The model under review builds one solid part; all positions refer to its coordinate system, in mm. Give positions to 0.01 mm unless a question says otherwise; leave off trailing zeros. Write each loop counter-clockwise with the first axis right and the second up, starting at its lowest first coordinate (ties: lowest second). Pieces come first, ordered by that corner, then holes. Notation, with made-up numbers: M 75,62 L 128,62 A14 cw 128,82 Z; hole C 83.25,72 d10. An arc over 180 degrees is marked long. Write item = value, one per line. Start each with the question number.
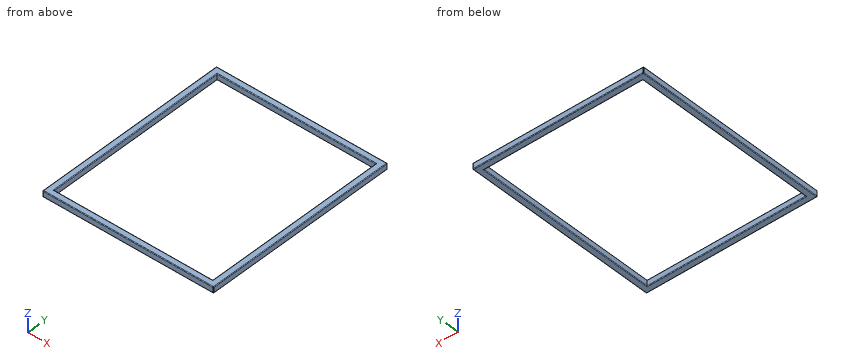
```python
from build123d import *

# Parameters (mm, degrees)
SKETCH1_W           = 711.2
SKETCH1_H           = 812.8
SKETCH1_W_2         = 660.4
SKETCH1_H_2         = 762
BOSS_EXTRUDE1_DEPTH = 25.4
FILLET1_R           = 2.54


with BuildPart() as part:
    # Sketch1 → Boss-Extrude1 (new body)
    with BuildSketch(Plane.XY):
        with Locations((-355.6, 406.4)):
            Rectangle(SKETCH1_W, SKETCH1_H)
        with Locations((-355.6, 406.4)):
            Rectangle(SKETCH1_W_2, SKETCH1_H_2, mode=Mode.SUBTRACT)
    extrude(amount=BOSS_EXTRUDE1_DEPTH)

    # Fillet1
    fillet1_edges = [part.edges().sort_by_distance(p)[0] for p in [
        (-711.2, 406.4, 25.4),
        (-25.4, 406.4, 0),
        (-355.6, 787.4, 0),
        (-685.8, 406.4, 0),
        (-355.6, 25.4, 0),
        (-25.4, 406.4, 25.4),
        (-355.6, 0, 25.4),
        (-355.6, 787.4, 25.4),
        (-685.8, 406.4, 25.4),
        (-355.6, 25.4, 25.4),
        (0, 406.4, 25.4),
        (-355.6, 0, 0),
        (-711.2, 406.4, 0),
        (-355.6, 812.8, 0),
        (0, 406.4, 0),
        (0, 0, 12.7),
        (-711.2, 0, 12.7),
        (-711.2, 812.8, 12.7),
        (0, 812.8, 12.7),
        (-355.6, 812.8, 25.4),
    ]]
    fillet(fillet1_edges, radius=FILLET1_R)


solid = part.part
```
Item 1: To check wall thickness, follow probe 1 along X at (y, z) = (775.5, 9.5); probe 2 along Y at (x, z) = (-496, 10.75); probe 3 along X at (y, z) = (487, 1.5). State the ranges of each line that lie inside material, in increasing order. Write a range as [from, to].
Item 2: We need section A-A, the plane x = -262. Write out the cut boundary in (y, z).
Item 3: We need section C-C, the plane z = 15. Write out the cut boundary in (x, y), and give its area (3 significant figures).
Item 4: We need section B-B, the plane y = 362. Write out the cut boundary in (x, z).
Worked out:
q1.probe_1 = [-711.2, -685.8], [-25.4, 0]
q1.probe_2 = [0, 25.4], [787.4, 812.8]
q1.probe_3 = [-710.98, -686.02], [-25.18, -0.22]
q2.outline = M 0,2.54 A2.54 ccw 2.54,0 L 22.86,0 A2.54 ccw 25.4,2.54 L 25.4,22.86 A2.54 ccw 22.86,25.4 L 2.54,25.4 A2.54 ccw 0,22.86 Z; M 787.4,2.54 A2.54 ccw 789.94,0 L 810.26,0 A2.54 ccw 812.8,2.54 L 812.8,22.86 A2.54 ccw 810.26,25.4 L 789.94,25.4 A2.54 ccw 787.4,22.86 Z
q3.outline = M -711.2,2.54 A2.54 ccw -708.66,0 L -2.54,0 A2.54 ccw 0,2.54 L 0,810.26 A2.54 ccw -2.54,812.8 L -708.66,812.8 A2.54 ccw -711.2,810.26 Z; hole M -685.8,25.4 L -25.4,25.4 L -25.4,787.4 L -685.8,787.4 Z
q3.area = 74,800 mm²
q4.outline = M -711.2,2.54 A2.54 ccw -708.66,0 L -688.34,0 A2.54 ccw -685.8,2.54 L -685.8,22.86 A2.54 ccw -688.34,25.4 L -708.66,25.4 A2.54 ccw -711.2,22.86 Z; M -25.4,2.54 A2.54 ccw -22.86,0 L -2.54,0 A2.54 ccw 0,2.54 L 0,22.86 A2.54 ccw -2.54,25.4 L -22.86,25.4 A2.54 ccw -25.4,22.86 Z
